The listing builds one solid part. Answer for the finished solid, in the listing's coordinates (mm). A direction names the side the tool comes from. Coordinates: 2 decimals unless noted, no trailing zeros. Order: outer loops, then holes, each group sorted by start corner. A loop starts at its lowest first (then second) coordinate and runs counter-clockwise, first axis right, second up. Notation, with made-up numbers: (70, 66.5) -> (86, 66.5) arc R34 ccw to (86, 102.5) -> close; hole circle Ø5 at (47.25, 39.25). An arc over 180 degrees is marked (long way). Return JSON: item names as keys, results as strings.
from build123d import *

# Parameters (mm, degrees)
SKETCH_1_W          = 120
SKETCH_1_H          = 130
EXTRUDE_1_DEPTH     = 20
SKETCH_2_R          = 42.5
CUT_EXTRUDE_1_DEPTH = 13
SKETCH_4_W          = 50
SKETCH_4_H          = 20
EXTRUDE_2_DEPTH     = 5
FILLET_2_R          = 30
FILLET_3_R          = 30
SKETCH_5_R          = 3
CUT_EXTRUDE_2_DEPTH = 168.705098312


with BuildPart() as part:
    # 草图1 → 凸台-拉伸1 (new body)
    with BuildSketch(Plane.XY):
        Rectangle(SKETCH_1_W, SKETCH_1_H)
    extrude(amount=EXTRUDE_1_DEPTH)

    # 草图2 → 切除-拉伸1 (cut)
    with BuildSketch(Plane.XY.offset(20)):
        with Locations((0, 5)):
            Circle(SKETCH_2_R)
    extrude(amount=-CUT_EXTRUDE_1_DEPTH, mode=Mode.SUBTRACT)

    # 草图4 → 凸台-拉伸2 (add)
    with BuildSketch(Plane.XZ.offset(65)):
        with Locations((85, 10)):
            Rectangle(SKETCH_4_W, SKETCH_4_H)
    extrude_2 = extrude(amount=-EXTRUDE_2_DEPTH)

    # 圆角2
    fillet_2_edges = [part.edges().sort_by_distance(p)[0] for p in [
        (60, -60, 10),
    ]]
    fillet(fillet_2_edges, radius=FILLET_2_R)

    # 镜向4: 凸台-拉伸2 across plane
    add(extrude_2.mirror(Plane(origin=(0, 0, 0), x_dir=(0, 0, 1), z_dir=(1, 0, 0))))

    # 圆角3
    fillet_3_edges = [part.edges().sort_by_distance(p)[0] for p in [
        (-60, -60, 10),
    ]]
    fillet(fillet_3_edges, radius=FILLET_3_R)

    # 草图5 → 切除-拉伸2 (cut, through all)
    with BuildSketch(Plane(origin=(0, -60, 0), x_dir=(1, 0, 0), z_dir=(0, 1, 0))):
        with Locations(Location((99.998041833, -10, 0), (0, 0, 270))):
            Circle(SKETCH_5_R)
    cut_extrude_2 = extrude(amount=-CUT_EXTRUDE_2_DEPTH, mode=Mode.SUBTRACT)

    # 镜向6: 切除-拉伸2 across plane
    add(cut_extrude_2.mirror(Plane(origin=(0, 0, 0), x_dir=(0, 0, 1), z_dir=(1, 0, 0))), mode=Mode.SUBTRACT)


solid = part.part
1. The part is cut by section C-C on y = 5. Give the vertices of the cut face in (x, z), and give its area (4 significant figures).
Answer block:
{"outline": "(-60, 0) -> (60, 0) -> (60, 20) -> (42.5, 20) -> (42.5, 7) -> (-42.5, 7) -> (-42.5, 20) -> (-60, 20) -> close", "area": "1,295 mm2"}
2. Consider line 1 (X direction, y = -61.05, z = 10); line 2 (X direction, y = 7, z = 13.25); line 3 (X direction, y = 6, z = 14.25). Determine where each line is inside the solid, lowest interval first. Write a range as from..to.
Answer block:
{"line 1": "x = -110..-103, -97..97, 103..110", "line 2": "x = -60..-42.45, 42.45..60", "line 3": "x = -60..-42.49, 42.49..60"}
3. The part is cut by section A-A on z = 10. Give the vertices of the cut face in (x, y), and give its area (3 significant figures).
Answer block:
{"outline": "(-110, -65) -> (-103, -65) -> (-103, -60) -> (-110, -60) -> close; (-97, -65) -> (97, -65) -> (97, -60) -> (90, -60) arc R30 cw to (60, -30) -> (60, 65) -> (-60, 65) -> (-60, -30) arc R30 cw to (-90, -60) -> (-97, -60) -> close; (103, -65) -> (110, -65) -> (110, -60) -> (103, -60) -> close; hole circle Ø85 at (0, 5)", "area": "10,800 mm2"}
4. Each of these flat-tipped pins is pushed along its axis until it touches: pin 1 Ø8 at (x, z) = (-100, 10) entering from +Y; pin 2 Ø1 at (y, z) = (-41, 12.5) entering from +X; pin 3 Ø10 at (y, z) = (37.5, 5) entering from +X. Where does it stop, or does it pass through?
Answer block:
{"pin 1": "stops at y = -60", "pin 2": "stops at x = 62.29", "pin 3": "stops at x = 60"}
5. The part is cut by section B-B on x = 0. Give the vertices of the cut face in (y, z), and give its area (4 significant figures).
Answer block:
{"outline": "(-65, 0) -> (65, 0) -> (65, 20) -> (47.5, 20) -> (47.5, 7) -> (-37.5, 7) -> (-37.5, 20) -> (-65, 20) -> close", "area": "1,495 mm2"}
6. Determine the mould class of faces 1 (the face through (60, 17, 10)), 2 (the face through (-60, 17, 10)), 3 (the face through (-9.21, -36.49, 13.59)) for opening direction X: pulls with the +X half, pulls with the -X half, needs draft (parallel to the pull), parting line crosses it, or undercut.
Answer block:
{"face 1": "pulls with the +X half", "face 2": "pulls with the -X half", "face 3": "undercut"}
7. The part is cut by section D-D on x = 66. Give the vertices of the cut face in (y, z).
Answer block:
{"outline": "(-65, 0) -> (-48, 0) -> (-48, 20) -> (-65, 20) -> close"}
8. For faces 4 (the face through (-97.6, -60, 12.4)), 5 (the face through (97.6, -60, 12.4)), 6 (the face through (-1, 6, 7)), determine the directions among +Z, -Z, +X, -X, +Y, -Y from which every point of the face is accessible in a straight line to the end or side of a thin tool.
Answer block:
{"face 4": "+Z, -Z, -X, +Y", "face 5": "+Z, -Z, +X, +Y", "face 6": "+Z"}
